CAD build for the part. Positions are in the model's coordinates, mm. Face numbers are marked on the shaded views. A direction names the side the tool comes from. Round coordinates to 2 decimals unless told otherwise and drop trailing zeros. Loops run counter-clockwise (first coordinate to the right, second up) from the corner with the lowest first, then second, coordinate; pieces in that order, holes last. Notation, with made-up numbers: M -39.75,-20 L -5.75,-20 A16 ccw -5.75,-1 Z; hole C 81,34.25 d8. An arc over 180 degrees is marked long. Use a Markdown table: item, result. Add a question column.
(1) Band-saw the part on B-B, the plane z = 4.5. Write the cut outline in (x, y).
(2) Which spindle directions (+Z, -Z, +X, -X, +Y, -Y) get a long thin tool onto all of the face, cutting with end or side? Do the marked faces 5 and 6. Say none if no direction does.
(3) Two-plate mould, pull along Y, no slides. Class the marked faces 1, 2, 3 and 4: released by +Y, released by -Y, zero draft, split by the parting line, or undercut.
(4) Band-saw the part on C-C, the plane y = 8.5. Write the cut outline in (x, z), and give its area (3 significant figures).
(5) Wall check: L1, parallel to Y at x = 0, z = 5.2; L2, parallel to Y at x = 2.5, z = 5.5; L3, parallel to Z at x = -11.5, y = 9.25. Give the ranges that are in metal, low to high.
(6) Band-saw the part on A-A, the plane x = 0. Write the cut outline in (y, z), and give its area (3 significant figures).
(7) Band-saw the part on D-D, the plane z = 9.5. Write the cut outline in (x, y).
(8) Flat gauge pins, fed straight in: P1, Ø4.5, axis at x = -18.25, y = 0, coming from the +Z side; P2, Ø6, axis at x = 4, z = 10.5, coming from the +Y side; P3, Ø5, axis at x = 12.5, z = 7.5, coming from the -Y side. Where does each tip first touch, or does it go through?
from build123d import *

# Parameters (mm, degrees)
BOSS_EXTRUDE5_DEPTH       = 4
SKETCH5_W                 = 2
SKETCH5_H                 = 4
F_5_0MM_DOWEL_HOLE1_D     = 5
F_5_0MM_DOWEL_HOLE1_DEPTH = 10.1
F_5_0MM_DOWEL_HOLE1_TIP   = 1.502151548
F_8_0MM_DOWEL_HOLE1_D     = 8
F_8_0MM_DOWEL_HOLE1_DEPTH = 10.1
F_8_0MM_DOWEL_HOLE1_TIP   = 2.403442476


with BuildPart() as part:
    # Sketch1 → Boss-Extrude5 (new body)
    with BuildSketch(Plane.XY):
        with BuildLine():
            Line((-20.660958904, 4.943407445), (-5.917808219, 12.133818273))
            ThreePointArc((-5.917808219, 12.133818273), (0, 13.5), (5.917808219, 12.133818273))
            Line((5.917808219, 12.133818273), (20.660958904, 4.943407445))
            ThreePointArc((20.660958904, 4.943407445), (23.75, 0), (20.660958904, -4.943407445))
            Line((20.660958904, -4.943407445), (5.917808219, -12.133818273))
            ThreePointArc((5.917808219, -12.133818273), (0, -13.5), (-5.917808219, -12.133818273))
            Line((-5.917808219, -12.133818273), (-20.660958904, -4.943407445))
            ThreePointArc((-20.660958904, -4.943407445), (-23.75, 0), (-20.660958904, 4.943407445))
        make_face()
    extrude(amount=BOSS_EXTRUDE5_DEPTH)

    # Sketch5 → Revolve2 (revolve)
    with BuildSketch(Plane(origin=(0, 0, 0), x_dir=(1, 0, 0), z_dir=(0, 1, 0)), mode=Mode.PRIVATE) as revolve2_sk:
        Polygon((4, -13), (6, -13), (6, -10.51697017), (6, -4), (4, -4), align=None)
        with Locations((12, -6)):
            Rectangle(SKETCH5_W, SKETCH5_H)
    revolve(revolve2_sk.sketch.rotate(Axis((0, 0, -13.433754879), (0, 0, 1)), 180), axis=Axis((0, 0, -13.433754879), (0, 0, 1)))

    # Ø5.0mm Dowel Hole1
    with Locations(Plane(origin=(0, 0, 0), x_dir=(1, 0, 0), z_dir=(0, 0, -1))):
        with Locations((18.25, 0), (-18.25, 0)):
            Hole(F_5_0MM_DOWEL_HOLE1_D / 2, depth=F_5_0MM_DOWEL_HOLE1_DEPTH)
            with Locations((0, 0, -(F_5_0MM_DOWEL_HOLE1_DEPTH + F_5_0MM_DOWEL_HOLE1_TIP / 2))):  # 118° drill point
                Cone(0, F_5_0MM_DOWEL_HOLE1_D / 2, F_5_0MM_DOWEL_HOLE1_TIP, mode=Mode.SUBTRACT)

    # Ø8.0mm Dowel Hole1
    with Locations(Plane.XY.offset(4)):
        with Locations((0, 0)):
            Hole(F_8_0MM_DOWEL_HOLE1_D / 2, depth=F_8_0MM_DOWEL_HOLE1_DEPTH)
            with Locations((0, 0, -(F_8_0MM_DOWEL_HOLE1_DEPTH + F_8_0MM_DOWEL_HOLE1_TIP / 2))):  # 118° drill point
                Cone(0, F_8_0MM_DOWEL_HOLE1_D / 2, F_8_0MM_DOWEL_HOLE1_TIP, mode=Mode.SUBTRACT)


solid = part.part
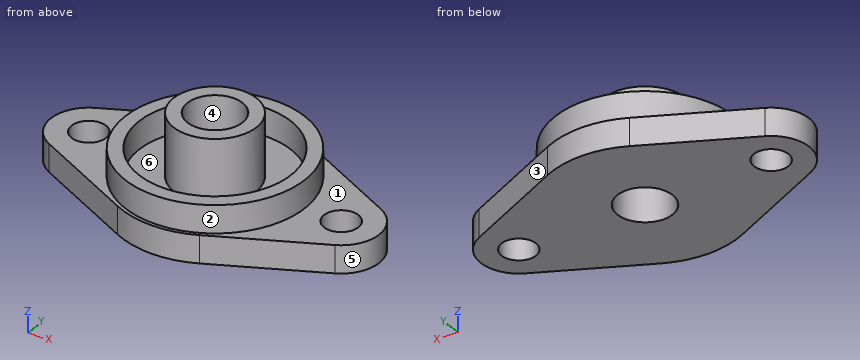
Return value:
| question | item | result |
|---|---|---|
| 1 | outline | C 0,0 d26; C 0,0 d12; hole C 0,0 d22; hole C 0,0 d8 |
| 2 | face 5 | +Z, -Z, +X |
| 2 | face 6 | +Z |
| 3 | face 1 | zero draft |
| 3 | face 2 | split by the parting line |
| 3 | face 3 | released by +Y |
| 3 | face 4 | undercut |
| 4 | outline | M -13.37,0 L 13.37,0 L 13.37,4 L 9.84,4 L 9.84,8 L 6.98,8 L 6.98,4 L -6.98,4 L -6.98,8 L -9.84,8 L -9.84,4 L -13.37,4 Z |
| 4 | area | 130 mm^2 |
| 5 | L1 | -13 to -11, -6 to -4, 4 to 6, 11 to 13 |
| 5 | L2 | -12.76 to -10.71, -5.45 to -3.12, 3.12 to 5.45, 10.71 to 12.76 |
| 5 | L3 | 0 to 4 |
| 6 | outline | M -13.5,0 L -4,0 L -4,13 L -6,13 L -6,4 L -11,4 L -11,8 L -13,8 L -13,4 L -13.5,4 Z; M 4,0 L 13.5,0 L 13.5,4 L 13,4 L 13,8 L 11,8 L 11,4 L 6,4 L 6,13 L 4,13 Z |
| 6 | area | 128 mm^2 |
| 7 | outline | C 0,0 d12; hole C 0,0 d8 |
| 8 | P1 | through |
| 8 | P2 | y = 12.79 |
| 8 | P3 | y = -8.31 |
